Work out the finished part from the listing and answer in its coordinate system (mm). A direction names the side the tool comes from. Coordinates: 2 decimals unless noted, no trailing zeros. Loops run counter-clockwise (first coordinate to the right, second up) from the corner with the lowest first, then second, coordinate; pieces in that order, holes last. Notation, with made-up numbers: (-26.5, 31.5) -> (11.5, 31.5) arc R11 cw to (11.5, 45.5) -> close; hole circle Ø1 at (22, 70.25). An arc over 180 degrees is marked (long way). Answer as CSV lines item,"result".
```python
from build123d import *

# Parameters (mm, degrees)
F0_W     = 609.6
F0_H     = 1219.2
F1_DEPTH = 1828.8
F2_W     = 1143
F2_H     = 44.45
F2_H_2   = 342.9
F2_H_3   = 381
F3_DEPTH = 2656.84
F4_W     = 533.4
F4_H     = 44.45
F4_H_2   = 342.9
F4_H_3   = 381
F5_DEPTH = 1470.66


with BuildPart() as f1:
    # F0 (on Top) → F1 (new body)
    with BuildSketch(Plane.XY):
        Rectangle(F0_W, F0_H)
    extrude(amount=F1_DEPTH)

    # F2 (on face) → F3 (cut)
    with BuildSketch(Plane.YZ.offset(304.8)):
        with Locations((0, 22.225)):
            Rectangle(F2_W, F2_H)
        with Locations((0, 292.1)):
            Rectangle(F2_W, F2_H_2)
        with Locations((0, 711.2)):
            Rectangle(F2_W, F2_H_2)
        with Locations((0, 1149.35)):
            Rectangle(F2_W, F2_H_3)
        with Locations((0, 1587.5)):
            Rectangle(F2_W, F2_H_2)
    extrude(amount=-F3_DEPTH, mode=Mode.SUBTRACT)

    # F4 (on face) → F5 (cut)
    with BuildSketch(Plane.XZ.offset(609.6)):
        with Locations((0, 22.225)):
            Rectangle(F4_W, F4_H)
        with Locations((0, 711.2)):
            Rectangle(F4_W, F4_H_2)
        with Locations((0, 292.1)):
            Rectangle(F4_W, F4_H_2)
        with Locations((0, 1149.35)):
            Rectangle(F4_W, F4_H_3)
        with Locations((0, 1587.5)):
            Rectangle(F4_W, F4_H_2)
    extrude(amount=-F5_DEPTH, mode=Mode.SUBTRACT)


solid = f1.part
```
(1) For a pull along Z with two mould halves and no side action, classify faces 6 (the face through (-266.7, 590, 22)), 7 (the face through (-285, -571.5, 709)), 8 (the face through (266.7, -591, 709)) as pulls with the +Z half, pulls with the -Z half, needs draft (parallel to the pull), parting line crosses it, or undercut.
Computed values:
face 6,"needs draft"
face 7,"undercut"
face 8,"undercut"
(2) Consider line 1 along Z through (x, y) = (121.5, 559); line 2 along Y through (x, z) = (-268, 708). Determine where each line is inside the solid, lowest interval first.
Computed values:
line 1,"44.45 to 120.65, 463.55 to 539.75, 882.65 to 958.85, 1339.85 to 1416.05, 1758.95 to 1828.8"
line 2,"-609.6 to -571.5, 571.5 to 609.6"
(3) A cutting plane is placed at C-C, the plane y = -289.5. Write down the section's boundary in (x, z), and give its area (3 significant figures).
Computed values:
outline,"(-304.8, 44.45) -> (304.8, 44.45) -> (304.8, 120.65) -> (-304.8, 120.65) -> close; (-304.8, 463.55) -> (304.8, 463.55) -> (304.8, 539.75) -> (-304.8, 539.75) -> close; (-304.8, 882.65) -> (304.8, 882.65) -> (304.8, 958.85) -> (-304.8, 958.85) -> close; (-304.8, 1339.85) -> (304.8, 1339.85) -> (304.8, 1416.05) -> (-304.8, 1416.05) -> close; (-304.8, 1758.95) -> (304.8, 1758.95) -> (304.8, 1828.8) -> (-304.8, 1828.8) -> close"
area,"228,000 mm2"
(4) Which of the six approach directions +Z, -Z, +X, -X, +Y, -Y give full straight-line access (tool end or side, diameter ignored) to faces 1 (the face through (266.7, -591, 290)), 2 (the face through (266.7, -591, 22)), 3 (the face through (-285, 571.5, 1147)), 4 (the face through (-285, 571.5, 22)), 5 (the face through (-72, 609.6, 495))?
Computed values:
face 1,"+Y, -Y"
face 2,"-Z, +Y, -Y"
face 3,"+X, -X"
face 4,"-Z, +X, -X"
face 5,"+Z, -Z, +X, -X, +Y"
(5) A cutting plane is placed at A-A, the plane x = -195. Write down the section's boundary in (y, z).
Computed values:
outline,"(-609.6, 44.45) -> (609.6, 44.45) -> (609.6, 120.65) -> (-609.6, 120.65) -> close; (-609.6, 463.55) -> (609.6, 463.55) -> (609.6, 539.75) -> (-609.6, 539.75) -> close; (-609.6, 882.65) -> (609.6, 882.65) -> (609.6, 958.85) -> (-609.6, 958.85) -> close; (-609.6, 1339.85) -> (609.6, 1339.85) -> (609.6, 1416.05) -> (-609.6, 1416.05) -> close; (-609.6, 1758.95) -> (609.6, 1758.95) -> (609.6, 1828.8) -> (-609.6, 1828.8) -> close"
(6) A flat-ended cylindrical pin translates along its axis: pin 1 Ø1.5 at (x, y) = (-127, 102.5) entering from -Z. Find the tip coordinate at first contact, or state that the pin passes through.
Computed values:
pin 1,"z = 44.45"
(7) A cutting plane is placed at B-B, the plane z = 1154. Write down the section's boundary in (x, y).
Computed values:
outline,"(-304.8, -609.6) -> (-266.7, -609.6) -> (-266.7, -571.5) -> (-304.8, -571.5) -> close; (-304.8, 571.5) -> (-266.7, 571.5) -> (-266.7, 609.6) -> (-304.8, 609.6) -> close; (266.7, -609.6) -> (304.8, -609.6) -> (304.8, -571.5) -> (266.7, -571.5) -> close; (266.7, 571.5) -> (304.8, 571.5) -> (304.8, 609.6) -> (266.7, 609.6) -> close"
